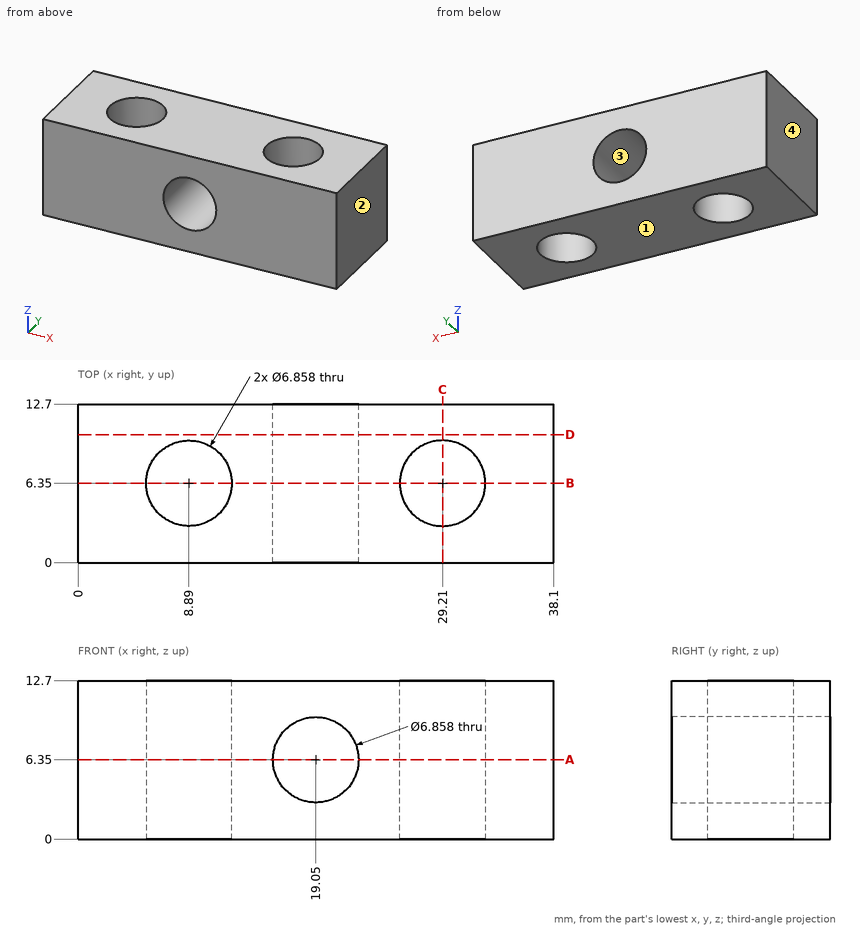
Geometry: see drawing. Coordinates: mm, zero at the bounding-box minimum. Coordinates: 2 decimals unless noted, no trailing zeros. Write each loop counter-clockwise with the first axis right and the second up, starting at its lowest first coordinate (ties: lowest second). Pieces come first, ordered by that corner, then holes. Notation, with made-up numbers: M 70.25,56 L 90.25,56 A26 ccw 90.25,82 Z; hole C -33.75,-18.5 d7. An arc over 180 degrees is marked long. Use CSV: the item, a comma, the result in double quotes. Start each with the question number.
1. Cut plane B-B on y = 6.35. Return the cut outline in (x, z), plus the area to 3 significant figures.
2. Cut plane C-C on x = 29.21. Return the cut outline in (y, z), plus the area to 3 significant figures.
3. Ray query, probe 1 along X at (y, z) = (5.75, 10); probe 2 along X at (y, z) = (5.25, 2); probe 3 along Y at (x, z) = (29.21, 8.75). Return the intervals inside material, ascending.
4. Cut plane D-D on y = 10.25. Return the cut outline in (x, z).
5. Mould query, pull axis X, two halves, no side actions, for the marked faces 1, 2, 3 and 4. Classes: pulls with the +X half, pulls with the -X half, needs draft (parallel to the pull), parting line crosses it, or undercut.
6. Cut plane A-A on z = 6.35. Return the cut outline in (x, y).
7. First-contact query: P1, Ø6, axis at y = 10.5, z = 3, coming from the -X side; P2, Ø5.5, axis at x = 29.21, y = 6.35, coming from the -Z side. Flat tips, straight axial feed; report the tip coordinate or a pass-through.
Entries:
1,outline,"M 0,0 L 5.46,0 L 5.46,12.7 L 0,12.7 Z; M 12.32,0 L 25.78,0 L 25.78,12.7 L 12.32,12.7 Z; M 32.64,0 L 38.1,0 L 38.1,12.7 L 32.64,12.7 Z; hole C 19.05,6.35 d6.86"
1,area,"273 mm²"
2,outline,"M 0,0 L 2.92,0 L 2.92,12.7 L 0,12.7 Z; M 9.78,0 L 12.7,0 L 12.7,12.7 L 9.78,12.7 Z"
2,area,"74.2 mm²"
3,probe 1,"0 to 5.51, 12.27 to 25.83, 32.59 to 38.1"
3,probe 2,"0 to 5.64, 12.14 to 25.96, 32.46 to 38.1"
3,probe 3,"0 to 2.92, 9.78 to 12.7"
4,outline,"M 0,0 L 38.1,0 L 38.1,12.7 L 0,12.7 Z; hole C 19.05,6.35 d6.86"
5,face 1,"needs draft"
5,face 2,"pulls with the +X half"
5,face 3,"undercut"
5,face 4,"pulls with the -X half"
6,outline,"M 0,0 L 15.62,0 L 15.62,12.7 L 0,12.7 Z; M 22.48,0 L 38.1,0 L 38.1,12.7 L 22.48,12.7 Z; hole C 8.89,6.35 d6.86; hole C 29.21,6.35 d6.86"
7,P1,"x = 0"
7,P2,"through"
